Input: part model. Units: mm. Frame: model coordinates. A direction names the side the tool comes from. Give positions to 0.01 mm unless a question says otherwise; leave off trailing zeros. Order: outer loops, then holes, each group sorted by start corner. A loop starts at its lowest first (then second) coordinate and runs counter-clockwise, first axis right, second up. Notation, with made-up numbers: (-38, 64.25) - (4, 64.25) arc R19 ccw to (4, 88.25) - close; hole circle Ø5 at (-22, 28). An arc over 180 degrees is marked (long way). Use a Markdown table: item, result.
from build123d import *

# Parameters (mm, degrees)
PAD004_DEPTH    = 3
SKETCH006_W     = 5
SKETCH006_H     = 3
PAD005_DEPTH    = 3
SKETCH008_R     = 1.85
POCKET002_DEPTH = 3.001
POCKET009_DEPTH = 3.001
SKETCH019_R     = 1.6
POCKET012_DEPTH = 3.001


with BuildPart() as part:
    # Sketch005 → Pad004 (new body)
    with BuildSketch(Plane.XY):
        with BuildLine():
            ThreePointArc((14.751455, 2.719296), (0, 15), (-14.751455, 2.719296))
            Line((-14.751455, 2.719296), (-30, -80))
            Line((-30, -80), (30, -80))
            Line((30, -80), (14.751455, 2.719296))
        make_face()
    extrude(amount=PAD004_DEPTH)

    # Sketch006 → Pad005 (join)
    with BuildSketch(Plane.XY):
        with Locations((-23.5, -81.5)):
            Rectangle(SKETCH006_W, SKETCH006_H)
        with Locations((23.5, -81.5)):
            Rectangle(SKETCH006_W, SKETCH006_H)
    extrude(amount=PAD005_DEPTH)

    # Sketch008 (on Face13 of Pad005) → Pocket002 (cut, through all)
    with BuildSketch(Plane(origin=(0, 0, 0), x_dir=(1, 0, 0), z_dir=(0, 0, -1))):
        with Locations((0, -8.25)):
            Circle(SKETCH008_R)
        with Locations((0, 19.75)):
            Circle(SKETCH008_R)
        with BuildLine():
            ThreePointArc((-2.943534, 5.228346), (0, -6), (2.943534, 5.228346))
            ThreePointArc((2.943534, 5.228346), (0, 9.5), (-2.943534, 5.228346))
        make_face()
    extrude(amount=-POCKET002_DEPTH, mode=Mode.SUBTRACT)

    # Sketch016 (on Face2 of Pocket002) → Pocket009 (cut, through all)
    with BuildSketch(Plane(origin=(0, 0, 0), x_dir=(1, 0, 0), z_dir=(0, 0, -1))):
        Polygon((-1.6, 80), (1.6, 80), (1.6, 70), (2.75, 70), (2.75, 67.2), (1.6, 67.2), (1.6, 60), (-1.6, 60), (-1.6, 67.2), (-2.75, 67.2), (-2.75, 70), (-1.6, 70), align=None)
    extrude(amount=-POCKET009_DEPTH, mode=Mode.SUBTRACT)

    # Sketch019 (on Face4 of Pocket009) → Pocket012 (cut, through all)
    with BuildSketch(Plane.XY.offset(3)):
        with Locations((-13.203501, -15.36091)):
            Circle(SKETCH019_R)
        Polygon((-13.417342, -7.695124), (-12.329624, -1.794542), (-9.182647, -2.374659), (-10.270365, -8.275241), align=None)
        Polygon((-12.98966, -23.026696), (-16.136638, -22.446579), (-17.224356, -28.347161), (-14.077379, -28.927278), align=None)
    extrude(amount=-POCKET012_DEPTH, mode=Mode.SUBTRACT)


solid = part.part
1. Material intervals for line 1 along Y through (x, z) = (0, 1.15); line 2 along X through (y, z) = (-2.5, 0.65); line 3 along Y through (x, z) = (2, 0.4), sorted ascending.
Response:
| item | result |
|---|---|
| line 1 | y = -60 to -21.6, -17.9 to -9.5, 6 to 6.4, 10.1 to 15 |
| line 2 | x = -15.71 to -12.46, -9.21 to -5.45, 5.45 to 15.71 |
| line 3 | y = -80 to -70, -67.2 to -8.78, 5.66 to 14.87 |
2. Set-up query: faces 1 (the face through (-22.27, -38.06, 1.48)), 2 (the face through (-21, -82, 1)), 3 (the face through (-11.82, -7.99, 1.52)), 4 (the face through (-26, -82, 1)). Return all of +Z, -Z, +X, -X, +Y, -Y with unobstructed straight access to the full face (end or side cutting, diameter ignored); none if empty.
Response:
| item | result |
|---|---|
| face 1 | +Z, -Z, -X, +Y |
| face 2 | +Z, -Z, -Y |
| face 3 | +Z, -Z |
| face 4 | +Z, -Z, -X, -Y |
3. Section query C-C (z = 1.55). State how many separate pieces and enclosed holes the cut face has, then the cut area to 3 significant figures.
Response:
| item | result |
|---|---|
| separate pieces | 1 |
| enclosed holes | 6 |
| area | 3,730 mm^2 |
4. Section query A-A (y = -72). Return loops of the section in (x, z).
Response:
| item | result |
|---|---|
| outline | (-28.53, 0) - (-1.6, 0) - (-1.6, 3) - (-28.53, 3) - close; (1.6, 0) - (28.53, 0) - (28.53, 3) - (1.6, 3) - close |
5. Section query D-D (x = -22). Return loops of the section in (y, z).
Response:
| item | result |
|---|---|
| outline | (-83, 0) - (-36.6, 0) - (-36.6, 3) - (-83, 3) - close |
6. Pin query (flat end, axial travel): pin 1 (5 mm diameter, centred on x = 24, y = -42, fed in from +Z); pin 2 (0.6 mm diameter, centred on x = -2, z = 1.5, fed in from +Y); pin 3 (1.5 mm diameter, centred on x = -0.5, z = 1.5, fed in from -Y); pin 4 (1 mm diameter, centred on y = -38.5, z = 1.5, fed in from -X). Return the tip coordinate at first contact, or that it passes through.
Response:
| item | result |
|---|---|
| pin 1 | stops at z = 3 |
| pin 2 | stops at y = 14.9 |
| pin 3 | stops at y = -60 |
| pin 4 | stops at x = -22.44 |
7. Mould query, pull axis Y, two halves, no side actions, for faces 5 (the face through (-9.72, -5.28, 1.52)), 6 (the face through (26, -82, 1)), 7 (the face through (23, -83, 1)). Classes: pulls with the +Y half, pulls with the -Y half, needs draft (parallel to the pull), parting line crosses it, or undercut.
Response:
| item | result |
|---|---|
| face 5 | undercut |
| face 6 | needs draft |
| face 7 | pulls with the -Y half |
8. Section query B-B (y = -6.35). Return loops of the section in (x, z).
Response:
| item | result |
|---|---|
| outline | (-16.42, 0) - (-13.17, 0) - (-13.17, 3) - (-16.42, 3) - close; (-9.92, 0) - (-3.15, 0) - (-3.15, 3) - (-9.92, 3) - close; (3.15, 0) - (16.42, 0) - (16.42, 3) - (3.15, 3) - close |
